Autodesk Inventor part; units mm, degrees
ref_plane "YZ Plane" through (0, 0, 0) normal (1, 0, 0) x (0, 1, 0)
ref_plane "XZ Plane" through (0, 0, 0) normal (0, 1, 0) x (-1, 0, 0)
ref_plane "XY Plane" through (0, 0, 0) normal (0, 0, 1) x (1, 0, 0)
sketch "Esquisse1" plane through (0, 0, 0) normal (0, 1, 0) x (-1, 0, 0)
  line L0 (-22.5, 22.5) -> (22.5, 22.5)
  line L1 (22.5, 22.5) -> (22.5, -22.5)
  line L2 (22.5, -22.5) -> (-22.5, -22.5)
  line L3 (-22.5, -22.5) -> (-22.5, 22.5)
  line L4 (-22.5, 22.5) -> (22.5, -22.5) construction
  line L5 (22.5, 22.5) -> (-22.5, -22.5) construction
  line L6 (-32.5, 32.5) -> (32.5, 32.5)
  line L7 (32.5, 32.5) -> (32.5, -32.5)
  line L8 (32.5, -32.5) -> (-32.5, -32.5)
  line L9 (-32.5, -32.5) -> (-32.5, 32.5)
  line L10 (-32.5, 32.5) -> (32.5, -32.5) construction
  line L11 (32.5, 32.5) -> (-32.5, -32.5) construction
  point P0 (0, 0)
  dimension "d0" = 45
  dimension "d1" = 45
  dimension "d2" = 65
extrude "Extrusion1" add sketch "Esquisse1" along normal blind 20
sketch "Esquisse2" plane through (-32.5, 0, 32.5) normal (0, 0, 1) x (1, 0, 0)
  line L0 (10, 20) -> (55, 20)
  line L1 (37.5, 0) -> (27.5, 0)
  line L2 (27.5, 0) -> (27.5, 20)
  line L3 (27.5, 20) -> (37.5, 20)
  line L4 (37.5, 20) -> (37.5, 0)
  line L5 (37.5, 0) -> (27.5, 20) construction
  line L6 (27.5, 0) -> (37.5, 20) construction
  point P0 (32.5, 0)
  dimension "d6" = 10
extrude "Extrusion2" add sketch "Esquisse2" along normal blind 35
sketch "Esquisse3" plane through (5, 0, 32.5) normal (1, 0, 0) x (0, 0, -1)
  line L0 (-35, 0) -> (-35, 20)
  line L1 (0, 0) -> (0, 20)
  point P0 (32.5, 0)
  point P1 (-17.5, 10)
hole "Perçage1" at (5, 10, 50) direction (-1, 0, 0) diameter 5 end through all
mirror "Symétrie1" about plane through (0, 0, 0) normal (0, 0, 1) of "Extrusion2", "Perçage1"
ref_plane "Plan de construction1" through (0, 0, 0) normal (0, 0, 1) x (1, 0, 0)
properties part number "Support moteur pas a pas"
Work out the finished part from the listing and answer in its coordinate system (mm). A direction names the side the tool comes from. Coordinates: 2 decimals unless noted, no trailing zeros. Loops run counter-clockwise (first coordinate to the right, second up) from the corner with the lowest first, then second, coordinate; pieces in that order, holes last. Notation, with made-up numbers: (44.25, -23.5) -> (95.25, -23.5) arc R27 cw to (95.25, 10.5) -> close; hole circle Ø6 at (88.5, -21). An arc over 180 degrees is marked (long way). Answer as CSV lines item,"result".
1) The part is cut by section D-D (y = 4.25). Give the vertices of the cut face in (x, z), and give its area (3 significant figures).
A:
outline,"(-32.5, -32.5) -> (-5, -32.5) -> (-5, -67.5) -> (5, -67.5) -> (5, -32.5) -> (32.5, -32.5) -> (32.5, 32.5) -> (5, 32.5) -> (5, 67.5) -> (-5, 67.5) -> (-5, 32.5) -> (-32.5, 32.5) -> close; hole (-22.5, -22.5) -> (22.5, -22.5) -> (22.5, 22.5) -> (-22.5, 22.5) -> close"
area,"2,900 mm²"
2) The part is cut by section B-B (z = -50). Give the vertices of the cut face in (x, y), and give its area (3 significant figures).
A:
outline,"(-5, 0) -> (5, 0) -> (5, 7.5) -> (-5, 7.5) -> close; (-5, 12.5) -> (5, 12.5) -> (5, 20) -> (-5, 20) -> close"
area,"150 mm²"
3) For a pull along Z with two mould halves and no side action, classify faces 1 (the face through (0, 10, -22.5)), 2 (the face through (-19, 10, -32.5)), 3 (the face through (-19, 10, 32.5)) as released by +Z, released by -Z, zero draft, split by the parting line, or undercut.
A:
face 1,"undercut"
face 2,"released by -Z"
face 3,"released by +Z"
4) The part is cut by section A-A (x = 3). Give the vertices of the cut face in (y, z), and give its area (3 significant figures).
A:
outline,"(0, -67.5) -> (20, -67.5) -> (20, -22.5) -> (0, -22.5) -> close; (0, 22.5) -> (20, 22.5) -> (20, 67.5) -> (0, 67.5) -> close; hole circle Ø5 at (10, -50); hole circle Ø5 at (10, 50)"
area,"1,760 mm²"
5) Flat-ended cylindrical pins translate along their axes: pin 1 (6 mm diameter, centred on y = 10, z = -50, fed in from -X); pin 2 (2 mm diameter, centred on x = -26, y = 8, fed in from +Z); pin 3 (8 mm diameter, centred on y = 10, z = 50, fed in from +X). Find the tip coordinate at first contact, or state that the pin passes through.
A:
pin 1,"stops at x = -5"
pin 2,"stops at z = 32.5"
pin 3,"stops at x = 5"
6) Straight lines are drawn through the part: probe 1 along Z at (x, y) = (-1.5, 10); probe 2 along Z at (x, y) = (-18, 18.5); probe 3 along Y at (x, z) = (1, 50). For each, find the intervals that lie inside material, in ascending order.
A:
probe 1,"z = -67.5 to -52.5, -47.5 to -22.5, 22.5 to 47.5, 52.5 to 67.5"
probe 2,"z = -32.5 to -22.5, 22.5 to 32.5"
probe 3,"y = 0 to 7.5, 12.5 to 20"
7) For faces 4 (the face through (-5, 10, 46)), 5 (the face through (-5, 10, -46)), 6 (the face through (5, 10, 46)), 7 (the face through (22.5, 10, 0)), determine the directions among +Z, -Z, +X, -X, +Y, -Y from which every point of the face is accessible in a straight line to the end or side of a thin tool.
A:
face 4,"+Z, -X, +Y, -Y"
face 5,"-Z, -X, +Y, -Y"
face 6,"+Z, +X, +Y, -Y"
face 7,"+Y, -Y"
8) The part is cut by section C-C (x = 17). Give the vertices of the cut face in (y, z), and give its area (3 significant figures).
A:
outline,"(0, -32.5) -> (20, -32.5) -> (20, -22.5) -> (0, -22.5) -> close; (0, 22.5) -> (20, 22.5) -> (20, 32.5) -> (0, 32.5) -> close"
area,"400 mm²"
